The listing builds one solid part. Answer for the finished solid, in the listing's coordinates (mm). Round coordinates to 2 decimals unless told otherwise and drop trailing zeros. Write each loop counter-clockwise with the first axis right and the second up, starting at its lowest first coordinate (ties: lowest second). Pieces come first, ordered by that corner, then holes.
Item 1: Find section B-B on z = 0. Give the vertices of the cut face in (x, y).
Item 2: Find section C-C on y = 2.7. Give the vertices of the cut face in (x, z).
Item 3: Find the intervals of material crossed by probe 1 along X at (y, z) = (1.7, 37); probe 2 along X at (y, z) = (4.3, -18); probe 3 along Z at (x, y) = (-49, 4), in increasing order.
Item 4: This flat-tipped pin is pushed along its axis until it touches: pin 1 (1 mm diameter, centred on x = -2.5, y = 2, fed in from -Z). Where does it stop, or does it pass through?
Item 5: Find section D-D on x = 23.5. Give the vertices of the cut face in (y, z).
Item 6: Find section A-A on x = 0. Give the vertices of the cut face in (y, z).
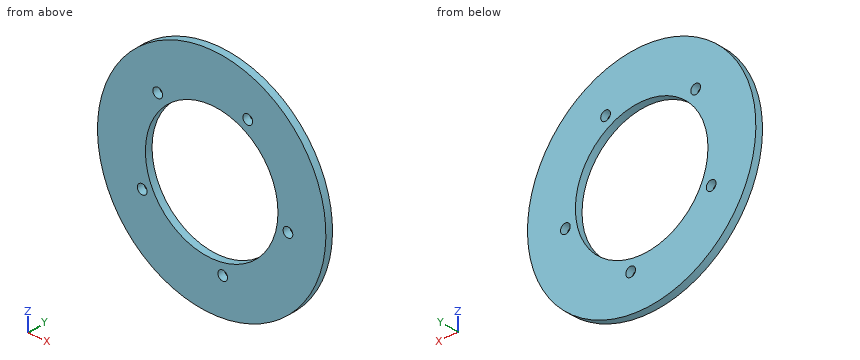
```python
from build123d import *

# Parameters (mm, degrees)
SKETCH1_R            = 77.5
SKETCH1_R_2          = 45
BODY_DEPTH           = 5
M6_CLEARANCE_HOLE1_D = 6.6


with BuildPart() as part:
    # Sketch1 → Body (new body)
    with BuildSketch(Plane(origin=(0, 0, 0), x_dir=(1, 0, 0), z_dir=(0, 1, 0))):
        with Locations(Location((0, 0, 0), (0, 0, 270))):
            Circle(SKETCH1_R)
        with Locations(Location((0, 0, 0), (0, 0, 270))):
            Circle(SKETCH1_R_2, mode=Mode.SUBTRACT)
    extrude(amount=BODY_DEPTH)

    # M6 Clearance Hole1 (through all)
    with Locations(Plane(origin=(0, 5, 0), x_dir=(1, 0, 0), z_dir=(0, 1, 0))):
        with Locations((7.5, 52), (51.772566305, 8.935959835), (24.497205661, -46.4772731), (-36.632460577, -37.660494315), (-47.13731139, 23.20180758), (0, 0)):
            Hole(M6_CLEARANCE_HOLE1_D / 2)


solid = part.part
```
Check values:
1. outline: (-77.5, 0) - (-45, 0) - (-45, 5) - (-77.5, 5) - close; (45, 0) - (77.5, 0) - (77.5, 5) - (45, 5) - close
2. outline: circle Ø155 at (0, 0); hole circle Ø6.6 at (-47.14, -23.2); hole circle Ø90 at (0, 0); hole circle Ø6.6 at (-36.63, 37.66); hole circle Ø6.6 at (7.5, -52); hole circle Ø6.6 at (24.5, 46.48); hole circle Ø6.6 at (51.77, -8.94)
3. probe 1: x = -68.1 to -39.87, -33.4 to -25.61, 25.61 to 68.1
3. probe 2: x = -75.38 to -41.24, 41.24 to 75.38
3. probe 3: z = -60.04 to -25.93, -20.48 to 60.04
4. pin 1: stops at z = -77.47
5. outline: (0, -73.85) - (5, -73.85) - (5, -38.38) - (0, -38.38) - close; (0, 38.38) - (5, 38.38) - (5, 43.33) - (0, 43.33) - close; (0, 49.62) - (5, 49.62) - (5, 73.85) - (0, 73.85) - close
6. outline: (0, -77.5) - (5, -77.5) - (5, -45) - (0, -45) - close; (0, 45) - (5, 45) - (5, 77.5) - (0, 77.5) - close
